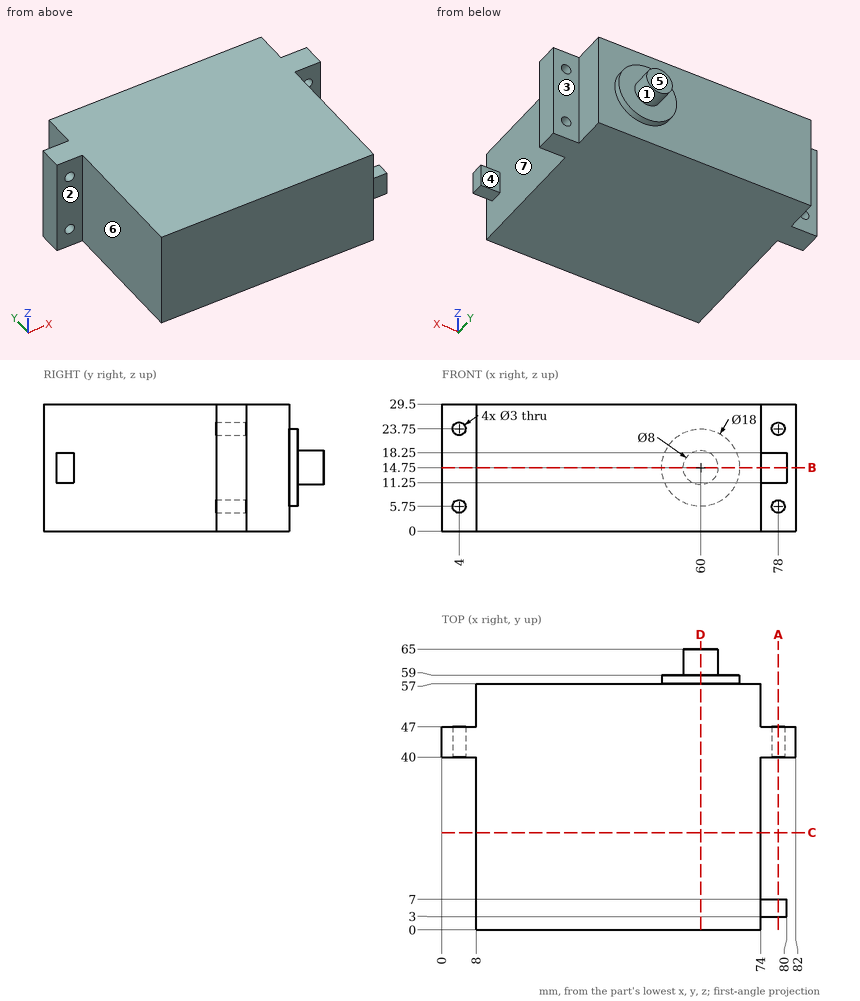
Source: three-view drawing plus pictorial views. Frame: mm from the lowest corner of the part. A direction names the side the tool comes from. Give positions to 0.01 mm unless a question says otherwise; leave off trailing zeros. Order: outer loops, then holes, each group sorted by start corner. A loop starts at its lowest first (then second) coordinate and runs counter-clockwise, first axis right, second up. Notation, with made-up numbers: M 11.5,43 L 54.5,43 A22 cw 54.5,55 Z; hole C 49,7 d2. An arc over 180 degrees is marked long. Return JSON: item names as keys, results as strings.
Item 1: Ray query, probe 1 along Z at (x, y) = (78, 42); probe 2 along X at (y, z) = (43, 23.75); probe 3 along Y at (x, z) = (15.5, 20.25). Return the intervals inside material, ascending.
Solutions:
{"probe 1": "0 to 4.25, 7.25 to 22.25, 25.25 to 29.5", "probe 2": "0 to 2.5, 5.5 to 76.5, 79.5 to 82", "probe 3": "0 to 57"}
Item 2: Cut plane C-C (y = 22.5). Return loops of the section in (x, z), then the cut area to 3 significant figures.
Solutions:
{"outline": "M 8,0 L 74,0 L 74,29.5 L 8,29.5 Z", "area": "1,950 mm^2"}
Item 3: Pull-direction query (Y, two-part tool) for the marked faces 4, 5, 6 and 7; classes: +Y half, -Y half, draft (parallel to the pull), parting line (faces both ways), or undercut.
Solutions:
{"face 4": "undercut", "face 5": "+Y half", "face 6": "draft", "face 7": "undercut"}
Item 4: First-contact query: P1, Ø1.2, axis at x = 76, y = 5, coming from the -Z side; P2, Ø3, axis at y = 5, z = 15, coming from the +X side; P3, Ø3, axis at x = 77.5, y = 5, coming from the +Z side. Flat tips, straight axial feed; report the tip coordinate or a pass-through.
Solutions:
{"P1": "z = 11.25", "P2": "x = 80", "P3": "z = 18.25"}
Item 5: Access query for the marked faces 1, 2 and 3. Directions: +Z, -Z, +X, -X, +Y, -Y. A direction counts if a zero-diameter tool reaches every point of the face in a straight line with its end or side. Return the directions, or none.
Solutions:
{"face 1": "+Y", "face 2": "+Z, -Z, -X, -Y", "face 3": "+Z, -Z, +X, +Y"}
Item 6: Cut plane A-A (x = 78). Return loops of the section in (y, z).
Solutions:
{"outline": "M 3,11.25 L 7,11.25 L 7,18.25 L 3,18.25 Z; M 40,0 L 47,0 L 47,4.25 L 40,4.25 Z; M 40,7.25 L 47,7.25 L 47,22.25 L 40,22.25 Z; M 40,25.25 L 47,25.25 L 47,29.5 L 40,29.5 Z"}
Item 7: Cut plane B-B (z = 14.75). Return loops of the section in (x, y), then the cut area to 3 significant figures.
Solutions:
{"outline": "M 0,40 L 8,40 L 8,0 L 74,0 L 74,3 L 80,3 L 80,7 L 74,7 L 74,40 L 82,40 L 82,47 L 74,47 L 74,57 L 69,57 L 69,59 L 64,59 L 64,65 L 56,65 L 56,59 L 51,59 L 51,57 L 8,57 L 8,47 L 0,47 Z", "area": "3,980 mm^2"}
Item 8: Cut plane D-D (x = 60). Return loops of the section in (y, z).
Solutions:
{"outline": "M 0,0 L 57,0 L 57,5.75 L 59,5.75 L 59,10.75 L 65,10.75 L 65,18.75 L 59,18.75 L 59,23.75 L 57,23.75 L 57,29.5 L 0,29.5 Z"}
